Autodesk Inventor part; units mm, degrees
ref_plane "YZ Plane" through (0, 0, 0) normal (1, 0, 0) x (0, 1, 0)
ref_plane "XZ Plane" through (0, 0, 0) normal (0, 1, 0) x (-1, 0, 0)
ref_plane "XY Plane" through (0, 0, 0) normal (0, 0, 1) x (1, 0, 0)
sketch "Sketch1" plane through (0, 0, 0) normal (0, 0, 1) x (1, 0, 0)
  line L0 (-12.7, -25.4) -> (12.7, -25.4)
  line L1 (12.7, -25.4) -> (12.7, 25.4)
  line L2 (12.7, 25.4) -> (-12.7, 25.4)
  line L3 (-12.7, 25.4) -> (-12.7, -25.4)
  line L4 (-12.7, -25.4) -> (12.7, 25.4) construction
  line L5 (12.7, -25.4) -> (-12.7, 25.4) construction
  line L6 (-11.1125, 23.8125) -> (11.1125, 23.8125)
  line L7 (11.1125, 23.8125) -> (11.1125, -23.8125)
  line L8 (11.1125, -23.8125) -> (-11.1125, -23.8125)
  line L9 (-11.1125, -23.8125) -> (-11.1125, 23.8125)
  point P0 (0, 0)
  dimension "width" = 25.4
  dimension "height" = 50.8
  dimension "thickness" = 1.5875
extrude "Extrusion1" add sketch "Sketch1" along normal mid plane 203.2
sketch "Sketch2" plane through (-12.7, 25.4, 101.6) normal (0, 1, 0) x (1, 0, 0)
  line L0 (0, 203.2) -> (0, 0) construction
  line L1 (25.4, 0) -> (0, 0) construction
  line L2 (25.4, 203.2) -> (25.4, 0) construction
  line L3 (0, 203.2) -> (25.4, 203.2) construction
  line L4 (12.7, 152.4) -> (12.7, 50.8) construction
  point P0 (12.7, 101.6)
  point P1 (12.7, 101.6)
  point P2 (12.7, 101.6)
  dimension "d5" = 101.6
hole "Hole1" at (0, 25.4, -50.8) at (0, 25.4, 50.8) at (0, 25.4, 0) direction (0, -1, 0) diameter 5.1054 end through all
sketch "Sketch4" plane through (12.7, -25.4, 101.6) normal (1, 0, 0) x (0, 0, -1)
  circle A0 centre (56.6109, 25.4) radius 53.75 construction
  line L0 (6.35, 6.35) -> (106.8718, 6.35) construction
  line L1 (106.8718, 6.35) -> (106.8718, 44.45) construction
  line L2 (106.8718, 44.45) -> (6.35, 44.45) construction
  line L3 (6.35, 44.45) -> (6.35, 6.35) construction
  line L4 (6.35, 6.35) -> (106.8718, 44.45) construction
  line L5 (106.8718, 6.35) -> (6.35, 44.45) construction
  line L6 (0, 0) -> (0, 50.8) construction
  point P0 (101.6, 25.4)
  dimension "d25" = 107.5
  dimension "d27" = 6.35
  dimension "d28" = 38.1
hole "Hole3" at (12.7, 19.05, 95.25) at (12.7, 19.05, -5.2718) at (12.7, -19.05, -5.2718) at (12.7, -19.05, 95.25) direction (-1, 0, 0) diameter 5.1054 end through all
sketch "Sketch3" plane through (12.7, -25.4, 101.6) normal (1, 0, 0) x (0, 0, -1)
  line L0 (51.3391, 44.45) -> (151.8609, 44.45) construction
  line L1 (151.8609, 44.45) -> (151.8609, 6.35) construction
  line L2 (151.8609, 6.35) -> (51.3391, 6.35) construction
  line L3 (51.3391, 6.35) -> (51.3391, 44.45) construction
  line L4 (51.3391, 44.45) -> (151.8609, 6.35) construction
  line L5 (151.8609, 44.45) -> (51.3391, 6.35) construction
  circle A0 centre (101.6, 25.4) radius 60 construction
  circle A1 centre (101.6, 25.4) radius 47.5 construction
  circle A2 centre (101.6, 25.4) radius 53.75 construction
  dimension "d16" = 107.5
  dimension "d14" = 120
  dimension "d15" = 95
  dimension "d17" = 38.1
properties part number "GP6-003" material "Aluminum 6061"
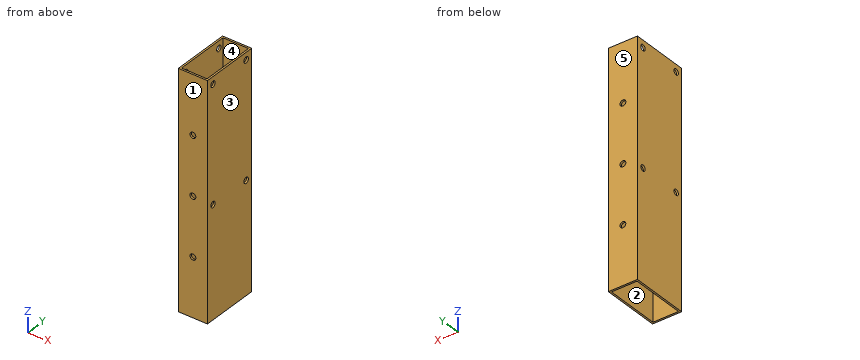
Here's how the part is built. I have some questions about the finished solid (model axes, mm). Face numbers are marked on the shaded views. A direction names the side the tool comes from. Give positions to 0.01 mm unless a question says otherwise; leave off trailing zeros. Loops run counter-clockwise (first coordinate to the right, second up) from the corner with the lowest first, then second, coordinate; pieces in that order, holes last. Notation, with made-up numbers: (-39.5, 39) -> (-3.5, 39) arc R14 cw to (-3.5, 52) -> close; hole circle Ø7 at (37, 84.5). An arc over 180 degrees is marked (long way). Answer as a JSON object with one key per item and string values. Group by question number.
Item 1: Imagine slicing it at D-D on z = 46.5. Write out the boundary of the cut face in (x, y), then the cut area to 3 significant figures.
Item 2: Imagine slicing it at A-A on y = 19.05. Write out the boundary of the cut face in (x, z).
Item 3: Imagine slicing it at C-C on x = -9. Write out the boundary of the cut face in (y, z), then the cut area to 3 significant figures.
Item 4: I need wall thicknesses on L1, parallel to Z at x = 0, y = -24.3; L2, parallel to Z at x = -11.9, y = 19.05; L3, parallel to Y at x = 12, z = 95.25. Which ranges of each line are inside material? Lowest first, please.
Item 5: On a 3-axis mill with a long thin cutter (end or side, diameter ignored), from which of +Z, -Z, +X, -X, +Y, -Y can I reach the whole of each face in a straight line? I mean the marked faces 4 and 5. Say none if no direction works.
Item 6: Imagine slicing it at B-B on z = 95.25. Write out the boundary of the cut face in (x, y).
Item 7: Thinking about a two-plate mould opening in X: for the marked faces 1, 2 and 3, which applies, pulls with the +X half, pulls with the -X half, needs draft (parallel to the pull), parting line crosses it, or undercut?
Answer list:
{
 "1": {"outline": "(-12.7, -25.4) -> (12.7, -25.4) -> (12.7, 25.4) -> (-12.7, 25.4) -> close; hole (-11.11, -23.81) -> (11.11, -23.81) -> (11.11, 23.81) -> (-11.11, 23.81) -> close", "area": "232 mm2"},
 "2": {"outline": "(-12.7, -101.6) -> (-11.11, -101.6) -> (-11.11, -7.82) -> (-12.7, -7.82) -> close; (-12.7, -2.72) -> (-11.11, -2.72) -> (-11.11, 92.7) -> (-12.7, 92.7) -> close; (-12.7, 97.8) -> (-11.11, 97.8) -> (-11.11, 101.6) -> (-12.7, 101.6) -> close; (11.11, -101.6) -> (12.7, -101.6) -> (12.7, -7.82) -> (11.11, -7.82) -> close; (11.11, -2.72) -> (12.7, -2.72) -> (12.7, 92.7) -> (11.11, 92.7) -> close; (11.11, 97.8) -> (12.7, 97.8) -> (12.7, 101.6) -> (11.11, 101.6) -> close"},
 "3": {"outline": "(-25.4, -101.6) -> (-23.81, -101.6) -> (-23.81, 101.6) -> (-25.4, 101.6) -> close; (23.81, -101.6) -> (25.4, -101.6) -> (25.4, 101.6) -> (23.81, 101.6) -> close", "area": "645 mm2"},
 "4": {"L1": "z = -101.6 to -53.35, -48.25 to -2.55, 2.55 to 48.25, 53.35 to 101.6", "L2": "z = -101.6 to -7.82, -2.72 to 92.7, 97.8 to 101.6", "L3": "y = -25.4 to -21.6, -16.5 to 16.5, 21.6 to 25.4"},
 "5": {"face 4": "+Z, -Z", "face 5": "+Z, -Z, +X, -X, +Y"},
 "6": {"outline": "(-12.7, -25.4) -> (12.7, -25.4) -> (12.7, -21.6) -> (11.11, -21.6) -> (11.11, -23.81) -> (-11.11, -23.81) -> (-11.11, -21.6) -> (-12.7, -21.6) -> close; (-12.7, -16.5) -> (-11.11, -16.5) -> (-11.11, 16.5) -> (-12.7, 16.5) -> close; (-12.7, 21.6) -> (-11.11, 21.6) -> (-11.11, 23.81) -> (11.11, 23.81) -> (11.11, 21.6) -> (12.7, 21.6) -> (12.7, 25.4) -> (-12.7, 25.4) -> close; (11.11, -16.5) -> (12.7, -16.5) -> (12.7, 16.5) -> (11.11, 16.5) -> close"},
 "7": {"face 1": "needs draft", "face 2": "undercut", "face 3": "pulls with the +X half"}
}
